Check sheet for the drawn part. Datum: minimum x, y, z corner. Units: mm. Round coordinates to 2 decimals unless told otherwise and drop trailing zeros. Order: outer loops, then holes, each group sorted by start corner. A loop starts at its lowest first (then second) coordinate and runs counter-clockwise, first axis right, second up. Notation, with made-up numbers: (-2, -23) -> (5, -23) arc R31 ccw to (5, 12) -> close; hole circle Ø6 at (44.25, -27.75). An arc over 180 degrees is marked (long way). Write item = value, one per line. Start each with the question number.
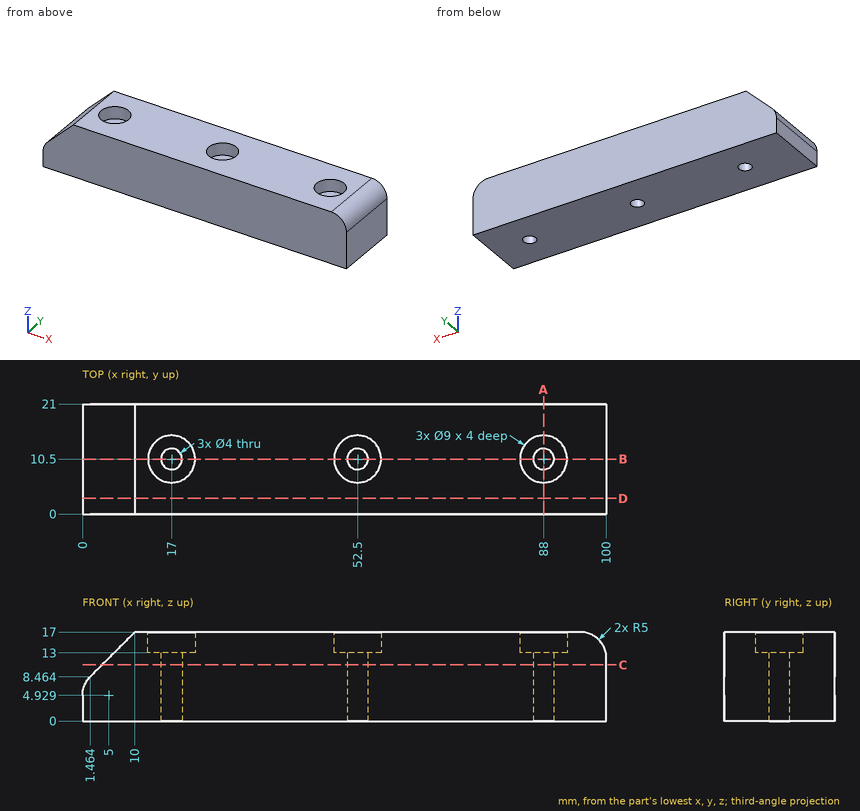
(1) Cross-section at D-D (y = 3). Enter the section's corners in (x, z) (1 decimal).
(2) Depth check by flat-ended pin: pin 1 (3 mm diameter, centred on y = 11, z = 15, fed in from -X); pin 2 (2.5 mm diameter, centred on x = 18.5, y = 11.5, fed in from +Z); pin 3 (2.5 mm diameter, centred on x = 17, y = 10.5, fed in from -Z); pin 4 (10 mm diameter, centred on y = 2.5, z = 11, fed in from -X). Enter the tip coordinate at first touch or a pass-through.
(3) Scan lines: line 1 along Y through (x, z) = (17, 14.85); line 2 along Y through (x, z) = (52.5, 8); line 3 along Z through (x, y) = (17.5, 7.5). Record each from-to range of solid material in increasing order. Write a range as from..to.
(4) Cross-section at C-C (z = 10.75). Enter the section's corners in (x, y), and give its area (3 significant figures).
(5) Cross-section at B-B (y = 10.5). Give the number of separate pieces and of enclosed holes in the cut face, and give its area (3 significant figures).
(6) Cross-section at A-A (x = 88). Enter the section's corners in (y, z), and give its area (3 significant figures).
Outcome:
q1.outline = (0, 0) -> (100, 0) -> (100, 12) arc R5 ccw to (95, 17) -> (10, 17) -> (1.5, 8.5) arc R5 ccw to (0, 4.9) -> close
q2.pin_1 = 6.5
q2.pin_2 = 13
q2.pin_3 = through
q2.pin_4 = 0.12
q3.line_1 = 0..6, 15..21
q3.line_2 = 0..8.5, 12.5..21
q3.line_3 = 0..13
q4.outline = (3.75, 0) -> (100, 0) -> (100, 21) -> (3.75, 21) -> close; hole circle Ø4 at (17, 10.5); hole circle Ø4 at (52.5, 10.5); hole circle Ø4 at (88, 10.5)
q4.area = 1,980 mm^2
q5.separate_pieces = 4
q5.enclosed_holes = 0
q5.area = 1,380 mm^2
q6.outline = (0, 0) -> (8.5, 0) -> (8.5, 13) -> (6, 13) -> (6, 17) -> (0, 17) -> close; (12.5, 0) -> (21, 0) -> (21, 17) -> (15, 17) -> (15, 13) -> (12.5, 13) -> close
q6.area = 269 mm^2
